Here's how the part is built. I have some questions about the finished solid (model axes, mm). A direction names the side the tool comes from. Coordinates: 2 decimals unless noted, no trailing zeros. Loops run counter-clockwise (first coordinate to the right, second up) from the corner with the lowest first, then second, coordinate; pieces in that order, holes last. Notation, with made-up numbers: M 23,40.5 L 64,40.5 A33 ccw 64,74.5 Z; hole C -34.5,12 d11. An arc over 180 degrees is marked long. Use CSV: the item, a comma, the result in double quotes. Start each with the question number.
Q1. If we mould it in two halves opening along Z, with no side actions, what happens to faces 1 (the flat face through (60.96, 13, -24)), 2 (the flat face through (120.607, 13, -3)), 3 (the flat face through (116.84, 12.52, -5.59)), 4 (the flat face through (67, 13, 9.536))? For each: +Z half, -Z half, draft (parallel to the pull), parting line (faces both ways), or undercut.
Q2. If we section it at B-B (x = 88): Please give me the cut outline in (y, z), and give its area (3 significant figures).
Q3. If we section it at C-C (z = -26): Please give me the cut outline in (x, y), and give its area (3 significant figures).
Q4. Please list where these lines run through material, in increasing order: probe 1 along Z at (x, y) = (-10, 14.25); probe 2 along X at (y, z) = (3.75, -5.5); probe 3 along Z at (x, y) = (84.5, 12.5). Write a range as [from, to].
Q5. Which directions (+Z, -Z, +X, -X, +Y, -Y) give clear straight access to the entire face, cutting with the end or side of a thin tool? Please do faces 5 (the flat face through (-36, 13, 5.798)), 6 (the flat face through (109, 13, -13.218)), 7 (the flat face through (-30, 13, -15.864)), 8 (the flat face through (109, 13, 7.102)).
Q6. For pin 1 Ø3 at (x, y) = (-18, 14) entering from +Z; pin 2 Ø8 at (x, z) = (16.5, 6) entering from -Y; pin 3 Ø1 at (x, y) = (95, 16.5) entering from -Z; pin 4 Ø1.9 at (y, z) = (7, 8) entering from -X, each with a flat end and sliding along its axis, tell me the tip position at first contact or that it passes through.
Q7. If we section it at A-A (y = 21.75): Please give me the cut outline in (x, z).
from build123d import *

# Parameters (mm, degrees)
F0_W     = 18.5124866861
F0_H     = 21.6614069645
F0_W_2   = 12.0454215246
F0_W_3   = 73.7178325796
F0_H_2   = 20.32
F1_DEPTH = 25.399999693
F2_R     = 5.08


with BuildPart() as f1:
    # F0 (on Front) → F1 (new body)
    with BuildSketch(Plane.XZ):
        with Locations((-60.7111408332, -5.0329225945)):
            Rectangle(F0_W, F0_H)
        Polygon((-74.0043607078, -11.8266495452), (-69.9673841763, -15.8636260767), (-69.9673841763, 5.7977808877), (-74.0043607078, 5.7977808877), align=None)
        with Locations((-45.4321867279, -5.0329225945)):
            Rectangle(F0_W_2, F0_H)
        Polygon((-39.4094759656, 5.7977808877), (-39.4094759656, -15.8636260767), (10.16, -15.8636260767), (10.16, 9.5363739233), (0, 9.5363739233), (0, 5.7977808877), align=None)
        Polygon((10.16, 9.5363739233), (10.16, -15.8636260767), (10.16, -31.1036260767), (20.1555099338, -31.1036260767), (20.1555099338, -15.7277081162), (31.0831721872, -15.5134415254), (31.0831721872, 9.3416357413), (19.0822575136, 9.3416357413), (19.0822575136, 24.7763739233), (10.16, 24.7763739233), align=None)
        Polygon((20.1555099338, -15.7277081162), (20.1555099338, -31.1036260767), (51.8696520655, -31.1036260767), (51.8696520655, -15.7424807711), (42.6536388695, -15.7424807711), (42.6536388695, 9.1273672879), (51.652893424, 9.3416357413), (51.652893424, 24.7763739233), (19.0822575136, 24.7763739233), (19.0822575136, 9.3416357413), (31.0831721872, 9.3416357413), (31.0831721872, -15.5134415254), align=None)
        Polygon((51.8696520655, -15.7424807711), (51.8696520655, -31.1036260767), (60.96, -31.1036260767), (60.96, -15.8636260767), (60.96, 9.5363739233), (60.96, 24.7763739233), (51.652893424, 24.7763739233), (51.652893424, 9.3416357413), (42.6536388695, 9.1273672879), (42.6536388695, -15.7424807711), align=None)
        Polygon((60.96, 9.5363739233), (60.96, -15.8636260767), (73.1124170143, -15.8636260767), (73.1124170143, -13.2178157567), (73.1124170143, 7.1021842433), (73.1124170143, 9.5363739233), align=None)
        with Locations((109.971333304, -3.0578157567)):
            Rectangle(F0_W_3, F0_H_2)
        Polygon((112.9683130925, -3.0190604849), (120.6068721646, 2.0565357327), (120.6068721646, -8.0946567025), align=None, mode=Mode.SUBTRACT)
    extrude(amount=-F1_DEPTH)

    # F2
    f2_edges = [f1.edges().sort_by_distance(p)[0] for p in [
        (10.16, 12.7, 24.776374),
    ]]
    fillet(f2_edges, radius=F2_R)


solid = f1.part
Results below:
1,face 1,"draft"
1,face 2,"undercut"
1,face 3,"undercut"
1,face 4,"+Z half"
2,outline,"M 0,-13.22 L 25.4,-13.22 L 25.4,7.1 L 0,7.1 Z"
2,area,"516 mm^2"
3,outline,"M 10.16,0 L 60.96,0 L 60.96,25.4 L 10.16,25.4 Z"
3,area,"1,290 mm^2"
4,probe 1,"[-15.86, 5.8]"
4,probe 2,"[-74, 116.7], [120.61, 146.83]"
4,probe 3,"[-13.22, 7.1]"
5,face 5,"+Z, -X, +Y, -Y"
5,face 6,"-Z, +X, +Y, -Y"
5,face 7,"-Z, -X, +Y, -Y"
5,face 8,"+Z, +X, +Y, -Y"
6,pin 1,"z = 5.8"
6,pin 2,"y = 0"
6,pin 3,"z = -13.22"
6,pin 4,"x = 0"
7,outline,"M -74,-11.83 L -69.97,-15.86 L 10.16,-15.86 L 10.16,-31.1 L 60.96,-31.1 L 60.96,-15.86 L 73.11,-15.86 L 73.11,-13.22 L 146.83,-13.22 L 146.83,7.1 L 73.11,7.1 L 73.11,9.54 L 60.96,9.54 L 60.96,24.78 L 15.24,24.78 A5.08 ccw 10.16,19.7 L 10.16,9.54 L 0,9.54 L 0,5.8 L -74,5.8 Z; hole M 112.97,-3.02 L 120.61,-8.09 L 120.61,2.06 Z"
